Autodesk Inventor part; units mm, degrees
ref_plane "YZ Plane" through (0, 0, 0) normal (1, 0, 0) x (0, 1, 0)
ref_plane "XZ Plane" through (0, 0, 0) normal (0, 1, 0) x (-1, 0, 0)
ref_plane "XY Plane" through (0, 0, 0) normal (0, 0, 1) x (1, 0, 0)
sketch "Sketch1" plane through (0, 0, 0) normal (0, 1, 0) x (-1, 0, 0)
  line L0 (0, 0) -> (-101.6, 0)
  line L1 (-101.6, 0) -> (-101.6, 457.2)
  line L2 (-101.6, 457.2) -> (0, 457.2)
  line L3 (0, 457.2) -> (0, 0)
  point P0 (-50.8, 228.6)
  dimension "d0" = 101.6
  dimension "d1" = 457.2
  dimension "d25" = 50.8
  dimension "d26" = 228.6
extrude "Extrusion1" add sketch "Sketch1" along normal blind 3.175
sketch "Sketch2" plane through (0, 3.175, 0) normal (0, 1, 0) x (1, 0, 0)
  line L0 (101.6, -457.2) -> (101.6, 0)
  line L1 (101.6, -457.2) -> (0, -457.2)
  line L2 (101.6, 0) -> (0, 0)
  point P0 (25.4, -12.7)
  point P1 (50.8, -12.7)
  point P2 (76.2, -12.7)
  point P3 (25.4, -444.5)
  point P4 (76.2, -444.5)
  point P5 (50.8, -444.5)
  dimension "d60" = 25.4
  dimension "d61" = 25.4
  dimension "d62" = 25.4
  dimension "d63" = 76.2
  dimension "d64" = 25.4
  dimension "d65" = 50.8
  dimension "d66" = 12.7
  dimension "d67" = 12.7
  dimension "d68" = 12.7
  dimension "d69" = 12.7
  dimension "d70" = 12.7
  dimension "d71" = 12.7
hole "Hole6" at (25.4, 3.175, 12.7) at (50.8, 3.175, 12.7) at (76.2, 3.175, 12.7) at (25.4, 3.175, 444.5) at (76.2, 3.175, 444.5) at (50.8, 3.175, 444.5) direction (0, -1, 0) diameter 6.35 end through all
sketch "Sketch3" plane through (0, 3.175, 0) normal (0, 1, 0) x (1, 0, 0)
  line L0 (0, 0) -> (0, -457.2)
  line L1 (101.6, -457.2) -> (101.6, 0)
  line L2 (101.6, 0) -> (0, 0)
  line L3 (0, -228.6) -> (101.6, -228.6)
  line L4 (101.6, 0) -> (101.6, -457.2)
  point P0 (69.85, -152.4)
  point P1 (31.75, -152.4)
  point P2 (31.75, -171.45)
  point P3 (69.85, -171.45)
  point P4 (69.85, -152.4)
  point P5 (31.75, -304.8)
  point P6 (31.75, -285.75)
  point P7 (69.85, -285.75)
  point P8 (69.85, -304.8)
  dimension "d79" = 38.1
  dimension "d80" = 19.05
  dimension "d81" = 31.75
  dimension "d82" = 31.75
  dimension "d83" = 152.4
  dimension "d84" = 19.05
  dimension "d85" = 38.1
  dimension "d86" = 152.4
hole "Hole7" at (69.85, 3.175, 152.4) at (31.75, 3.175, 152.4) at (31.75, 3.175, 171.45) at (69.85, 3.175, 171.45) at (31.75, 3.175, 285.75) at (31.75, 3.175, 304.8) at (69.85, 3.175, 304.8) at (69.85, 3.175, 285.75) direction (0, -1, 0) diameter 6.35 end through all
sketch "Sketch4" plane through (0, 3.175, 0) normal (0, 1, 0) x (1, 0, 0)
  line L0 (0, 0) -> (0, -457.2)
  line L1 (101.6, 0) -> (0, 0)
  point P0 (50.8, -163.5125)
  point P1 (50.8, -293.6875)
  dimension "d94" = 130.175
  dimension "d95" = 50.8
  dimension "d96" = 50.8
  dimension "d97" = 163.5125
hole "Hole8" at (50.8, 3.175, 163.5125) at (50.8, 3.175, 293.6875) direction (0, -1, 0) diameter 6.35 end through all
properties part number "Claw Plate"
CAD build for the part. Positions are in the model's coordinates, mm. Round coordinates to 2 decimals unless told otherwise and drop trailing zeros.
Item 1: Drop flat-ended pins along their axis: pin 1 Ø8 at (x, z) = (83, 85) entering from -Y; pin 2 Ø4 at (x, z) = (76.2, 444.5) entering from +Y. Give the stop position or say it passes through.
Filled in:
pin 1: stops at y = 0
pin 2: passes through
Item 2: Mould opens along Y. For faces 1 (the flat face through (52, 0, 232)), 2 (the flat face through (52, 3.175, 232)) say: released by +Y, released by -Y, zero draft, split by the parting line, or undercut.
Filled in:
face 1: released by -Y
face 2: released by +Y
Item 3: Drill centre lines: L1, parallel to Z at x = 69.85, y = 2.25 (3 decimals); L2, parallel to Z at x = 70.5, y = 1.6; L3, parallel to X at y = 0.75, z = 304.8 (3 decimals). Where is each one in solid material? Low to high.
Filled in:
L1: z = 0 to 149.225, 155.575 to 168.275, 174.625 to 282.575, 288.925 to 301.625, 307.975 to 457.2
L2: z = 0 to 149.29, 155.51 to 168.34, 174.56 to 282.64, 288.86 to 301.69, 307.91 to 457.2
L3: x = 0 to 28.575, 34.925 to 66.675, 73.025 to 101.6
